Autodesk Inventor part; units mm, degrees
ref_plane "YZ Plane" through (0, 0, 0) normal (1, 0, 0) x (0, 1, 0)
ref_plane "XZ Plane" through (0, 0, 0) normal (0, 1, 0) x (-1, 0, 0)
ref_plane "XY Plane" through (0, 0, 0) normal (0, 0, 1) x (1, 0, 0)
ref_plane "Work Plane1" through (-420.2595, 673.9641, 1040.2284) normal (0, 1, 0) x (-1, 0, 0)
sketch "Sketch1" plane through (-420.2595, 673.9641, 1040.2284) normal (0, 1, 0) x (-1, 0, 0)
  line L0 (-1974.87, 175.87) -> (-25.13, 175.87) construction
  line L1 (-25.13, -175.87) -> (-1974.87, -175.87) construction
  line L2 (-24.13, 0) -> (-24.13, 224.13) construction
  line L3 (-1975.87, -224.13) -> (-1975.87, 0) construction
  line L4 (-1975.87, 0) -> (-1975.87, 224.13) construction
  line L5 (-24.13, -224.13) -> (-24.13, 0) construction
  line L6 (-300, 175.87) -> (-1700, 175.87)
  line L7 (-1700, 175.87) -> (-1700, -175.87)
  line L8 (-1700, -175.87) -> (-300, -175.87)
  line L9 (-300, -175.87) -> (-300, 175.87)
  point P0 (-420.2595, -1040.2284)
  point P1 (-1000, 175.87)
  point P2 (-1000, -175.87)
  point P3 (-1000, -175.87)
  dimension "d0" = 1400
extrude "Plate1" add sketch "Sketch1" along normal blind 3.048
sketch "Sketch2" plane through (1276.6925, 673.9641, 864.3584) normal (1, 0, 0) x (0, 1, 0)
  line L0 (0, 351.74) -> (0, 0)
  line L1 (0, 0) -> (300, 0)
  line L2 (300, 0) -> (300, 351.74)
  line L3 (300, 351.74) -> (0, 351.74)
edge flange "Flange1" height 300 angle 90 thickness 3.048 bend radius 3.048 thickness toward (1, 0, 0) relief tear relief width 3.048 relief depth 1.524 corner gap 3.048 corner form 0 edges at (1279.7405, 677.0121, 1040.2284) (-120.2595, 677.0121, 1040.2284) wall of the first edge with corners at (1276.6925, 673.9641, 1216.0984) (1276.6925, 673.9641, 864.3584) (1276.6925, 973.9641, 864.3584) (1276.6925, 973.9641, 1216.0984)
bend "Bend1"
corner "Corner1"
fillet "Corner Round1" radius 120 4 edges at (-118.7355, 973.9641, 1216.0984) (-118.7355, 973.9641, 864.3584) (1278.2165, 973.9641, 1216.0984) (1278.2165, 973.9641, 864.3584)
equation "\"d1\" = Thickness"
equation "\"d2\" = BendReliefWidth"
equation "\"d3\" = BendReliefDepth"
equation "\"d4\" = MinimumRemnant"
equation "\"d5\" = TransitionRadius"
equation "\"d8\" = BendRadius"
equation "\"d9\" = CornerReliefSize"
equation "\"d10\" = GapSize"
equation "\"d11\" = JacobiRadiusSize"
equation "\"BendRadius\" = Thickness"
equation "\"BendReliefWidth\" = Thickness"
equation "\"BendReliefDepth\" = 0.5 * Thickness"
equation "\"CornerReliefSize\" = 4 * Thickness"
equation "\"MinimumRemnant\" = 2 * Thickness"
equation "\"TransitionRadius\" = BendRadius"
equation "\"JacobiRadiusSize\" = BendRadius"
equation "\"GapSize\" = Thickness"
properties part number "CE-5.2.3-03"
Read the model definition and answer for the solid it produces. Units are mm, in the model's axes. A direction names the side the tool comes from. Coordinates: 2 decimals unless noted, no trailing zeros. Write each loop counter-clockwise with the first axis right and the second up, starting at its lowest first coordinate (ties: lowest second). Pieces come first, ordered by that corner, then holes. Notation, with made-up numbers: (30, -30.5) - (49, -30.5) arc R16 cw to (49, -7.5) - close; hole circle Ø6 at (25.25, 70). An arc over 180 degrees is marked (long way). Answer as a JSON object with one key per item and string values. Group by question number.
1. A cutting plane is placed at C-C (x = 784). Determine the outline of the cut face in (y, z), plus the area to 3 significant figures.
2. Which of the six approach directions +Z, -Z, +X, -X, +Y, -Y give full straight-line access (tool end or side, diameter ignored) to faces 1 (the flat face through (1279.74, 829, 1038)), 2 (the flat face through (-117.212, 825, 1043))?
3. A cutting plane is placed at A-A (y = 770). Determine the outline of the cut face in (x, z), plus the area to 3 significant figures.
4. Consider L1, parallel to X at y = 927.5, z = 1129.5; L2, parallel to Y at x = 680, z = 1050. Determine where each line is inside the solid, lowest interval first. Write a range as [from, to].
5. The mould has two halves that part along X. Classify faces 3 (the flat face through (-120.26, 829, 1043)), 4 (the cylindrical face through (1278.238, 939.745, 1180.013)), 5 (the flat face through (1276.692, 825, 1038)): +X half, -X half, draft (parallel to the pull), parting line (faces both ways), or undercut.
6. A cutting plane is placed at D-D (y = 927.5). Determine the outline of the cut face in (x, z), plus the area to 3 significant figures.
7. This flat-tipped pin is pushed along its axis until it touches: P1, Ø1.5, axis at x = 710.5, z = 1026, coming from the +Y side. Where does it stop, or does it pass through?
8. A cutting plane is placed at B-B (z = 1167.5). Determine the outline of the cut face in (x, y).
Worked out:
{
 "1": {"outline": "(673.96, 864.36) - (677.01, 864.36) - (677.01, 1216.1) - (673.96, 1216.1) - close", "area": "1,070 mm²"},
 "2": {"face 1": "+Z, -Z, +X, +Y, -Y", "face 2": "+Z, -Z, +Y"},
 "3": {"outline": "(-120.26, 864.36) - (-117.21, 864.36) - (-117.21, 1216.1) - (-120.26, 1216.1) - close; (1276.69, 864.36) - (1279.74, 864.36) - (1279.74, 1216.1) - (1276.69, 1216.1) - close", "area": "2,140 mm²"},
 "4": {"L1": "x = [-120.26, -117.21], [1276.69, 1279.74]", "L2": "y = [673.96, 677.01]"},
 "5": {"face 3": "-X half", "face 4": "draft", "face 5": "undercut"},
 "6": {"outline": "(-120.26, 889.53) - (-117.21, 889.53) - (-117.21, 1190.93) - (-120.26, 1190.93) - close; (1276.69, 889.53) - (1279.74, 889.53) - (1279.74, 1190.93) - (1276.69, 1190.93) - close", "area": "1,840 mm²"},
 "7": {"P1": "stops at y = 677.01"},
 "8": {"outline": "(-120.26, 680.06) arc R6.1 ccw to (-114.16, 673.96) - (1273.64, 673.96) arc R6.1 ccw to (1279.74, 680.06) - (1279.74, 950.41) - (1276.69, 950.41) - (1276.69, 680.06) arc R3.05 cw to (1273.64, 677.01) - (-114.16, 677.01) arc R3.05 cw to (-117.21, 680.06) - (-117.21, 950.41) - (-120.26, 950.41) - close"}
}
